Build history of the part. All positions in model axes, mm. A direction names the side the tool comes from. Give positions to 0.01 mm unless a question says otherwise; leave off trailing zeros. Loops run counter-clockwise (first coordinate to the right, second up) from the corner with the lowest first, then second, coordinate; pieces in that order, holes last. Notation, with made-up numbers: (-15, 71.25) -> (-9, 71.25) arc R19 ccw to (-9, 100.25) -> close; hole circle Ø2 at (-27.5, 28.25). An arc over 180 degrees is marked (long way). One line per question, with ' | ' between items. Start each with the question number.
(1) Mould opens along X. For faces 5 (the face through (35.85, -4.68, 3.94)), 6 (the face through (-6.5, -32, 12)), 7 (the face through (37, 0, 21.9)), 8 (the face through (0, -32, 15.45)) say: pulls with the +X half, pulls with the -X half, needs draft (parallel to the pull), parting line crosses it, or undercut.
(2) Slice it at D-D, the plane x = -37.5. Write the cut outline in (y, z), then the cut area to 3 significant figures.
(3) Drill centre lines: L1, parallel to Y at x = 37.5, z = 4.25; L2, parallel to Y at x = 37.5, z = 22.6; L3, parallel to Y at x = -26.5, z = 8. Where is each one in solid material? Low to high. Write a range as from..to.
(4) Slice it at A-A, the plane z = 12. Write the cut outline in (x, y).
(5) Slice it at B-B, the plane x = 0. Write the cut outline in (y, z), then the cut area to 3 significant figures.
(6) Slice it at C-C, the plane y = 0. Write the cut outline in (x, z).
(7) Flat gauge pins, fed straight in: pin 1 Ø9 at (y, z) = (-28.5, 12) entering from -X; pin 2 Ø5.5 at (x, y) = (37.5, -4.75) entering from -Z; pin 3 Ø7 at (x, y) = (0, 0) entering from +Z; pin 4 Ø8 at (x, z) = (-12, 12) entering from -Y. Where does each tip first touch, or does it go through?
(8) 3-axis set-ups, long thin cutter, end or side, ignore diameter. For faces 1 (the face through (41.792, 1.352, 22.407)), 2 (the face through (-1, 10, 11)), 3 (the face through (-38, -5, 8)), 4 (the face through (6.5, -32, 12)): which of +Z, -Z, +X, -X, +Y, -Y reach the whole face in a straight line?
```python
from build123d import *

# Parameters (mm, degrees)
SK_BODY_W              = 97
SK_BODY_H              = 29.5
EX_BODY_DEPTH          = 22.9
SK_VESA_2XM4_R         = 1.65
CUT_VESA_2XM4_DEPTH    = 8
SK_LENSES_R            = 4.5
SK_LENSES_W            = 14
SK_LENSES_H            = 10
CUT_LENSES_DEPTH       = 1
SK_KEEPOUT_USB_C_W     = 13
SK_KEEPOUT_USB_C_H     = 8
EX_KEEPOUT_USB_C_DEPTH = 25


with BuildPart() as part:
    # SK_Body → EX_Body (new body)
    with BuildSketch(Plane.XY):
        with Locations((0, -4.75)):
            Rectangle(SK_BODY_W, SK_BODY_H)
    extrude(amount=EX_BODY_DEPTH)

    # SK_VESA_2xM4 → CUT_VESA_2xM4 (cut)
    with BuildSketch(Plane.XY):
        with Locations((37.5, -4.75)):
            Circle(SK_VESA_2XM4_R)
        with Locations((-37.5, -4.75)):
            Circle(SK_VESA_2XM4_R)
    extrude(amount=CUT_VESA_2XM4_DEPTH, mode=Mode.SUBTRACT)

    # SK_Lenses → CUT_Lenses (cut)
    with BuildSketch(Plane.XY.offset(22.9)):
        with Locations((37.5, 0)):
            Circle(SK_LENSES_R)
        with Locations((-37.5, 0)):
            Circle(SK_LENSES_R)
        Circle(SK_LENSES_R)
        with Locations((17, 0)):
            Rectangle(SK_LENSES_W, SK_LENSES_H)
    extrude(amount=-CUT_LENSES_DEPTH, mode=Mode.SUBTRACT)

    # SK_KeepOut_USB_C → EX_KeepOut_USB_C (add)
    with BuildSketch(Plane(origin=(0, -19.5, 0), x_dir=(1, 0, 0), z_dir=(0, 1, 0))):
        with Locations((0, -11.45)):
            Rectangle(SK_KEEPOUT_USB_C_W, SK_KEEPOUT_USB_C_H)
    extrude(amount=-EX_KEEPOUT_USB_C_DEPTH)


solid = part.part
```
Final values:
1) face 5: undercut | face 6: pulls with the -X half | face 7: undercut | face 8: needs draft
2) outline: (-19.5, 0) -> (-6.4, 0) -> (-6.4, 8) -> (-3.1, 8) -> (-3.1, 0) -> (10, 0) -> (10, 22.9) -> (4.5, 22.9) -> (4.5, 21.9) -> (-4.5, 21.9) -> (-4.5, 22.9) -> (-19.5, 22.9) -> close | area: 640 mm2
3) L1: -19.5..-6.4, -3.1..10 | L2: -19.5..-4.5, 4.5..10 | L3: -19.5..10
4) outline: (-48.5, -19.5) -> (-6.5, -19.5) -> (-6.5, -44.5) -> (6.5, -44.5) -> (6.5, -19.5) -> (48.5, -19.5) -> (48.5, 10) -> (-48.5, 10) -> close
5) outline: (-44.5, 7.45) -> (-19.5, 7.45) -> (-19.5, 0) -> (10, 0) -> (10, 22.9) -> (4.5, 22.9) -> (4.5, 21.9) -> (-4.5, 21.9) -> (-4.5, 22.9) -> (-19.5, 22.9) -> (-19.5, 15.45) -> (-44.5, 15.45) -> close | area: 867 mm2
6) outline: (-48.5, 0) -> (48.5, 0) -> (48.5, 22.9) -> (42, 22.9) -> (42, 21.9) -> (33, 21.9) -> (33, 22.9) -> (24, 22.9) -> (24, 21.9) -> (10, 21.9) -> (10, 22.9) -> (4.5, 22.9) -> (4.5, 21.9) -> (-4.5, 21.9) -> (-4.5, 22.9) -> (-33, 22.9) -> (-33, 21.9) -> (-42, 21.9) -> (-42, 22.9) -> (-48.5, 22.9) -> close
7) pin 1: x = -6.5 | pin 2: z = 0 | pin 3: z = 21.9 | pin 4: y = -19.5
8) face 1: +Z | face 2: +Z, -Z, +X, -X, +Y | face 3: -Z | face 4: +Z, -Z, +X, -Y
